from build123d import *

# Parameters (mm, degrees)
BOSS_EXTRUDE1_DEPTH = 3
SKETCH2_W           = 10
SKETCH2_H           = 3
SKETCH2_W_2         = 3
SKETCH2_H_2         = 12
CUT_EXTRUDE1_DEPTH  = 10
SKETCH5_R           = 1.7
SKETCH5_W           = 3
SKETCH5_H           = 5
CUT_EXTRUDE2_DEPTH  = 3
SKETCH6_R           = 2.5
SKETCH6_R_2         = 2.25
CUT_EXTRUDE3_DEPTH  = 10


with BuildPart() as part:
    # Sketch1 → Boss-Extrude1 (new body)
    with BuildSketch(Plane.XY.offset(152)):
        with BuildLine():
            Line((-82, 69.5), (82, 69.5))
            Line((82, 69.5), (82, 44))
            Line((82, 44), (88.6, 44))
            Line((88.6, 44), (88.6, 47))
            Line((88.6, 47), (93.6, 47))
            Line((93.6, 47), (93.6, 44))
            Line((93.6, 44), (98.6, 44))
            Line((98.6, 44), (98.6, 43.377104502))
            ThreePointArc((98.6, 43.377104502), (94.427800977, -13.668492876), (82, -69.5))
            Line((82, -69.5), (-82, -69.5))
            ThreePointArc((-82, -69.5), (-94.427800977, -13.668492876), (-98.6, 43.377104502))
            Line((-98.6, 43.377104502), (-98.6, 44))
            Line((-98.6, 44), (-93.6, 44))
            Line((-93.6, 44), (-93.6, 47))
            Line((-93.6, 47), (-88.6, 47))
            Line((-88.6, 47), (-88.6, 44))
            Line((-88.6, 44), (-82, 44))
            Line((-82, 44), (-82, 69.5))
        make_face()
    extrude(amount=BOSS_EXTRUDE1_DEPTH)

    # Sketch2 → Cut-Extrude1 (cut)
    with BuildSketch(Plane.XY.offset(155)):
        with Locations((0, 68)):
            Rectangle(SKETCH2_W, SKETCH2_H)
        with Locations((-22, 68)):
            Rectangle(SKETCH2_W, SKETCH2_H)
        with Locations((22, 68)):
            Rectangle(SKETCH2_W, SKETCH2_H)
        with Locations((-44, 68)):
            Rectangle(SKETCH2_W, SKETCH2_H)
        with Locations((44, 68)):
            Rectangle(SKETCH2_W, SKETCH2_H)
        with Locations((-66, 68)):
            Rectangle(SKETCH2_W, SKETCH2_H)
        with Locations((66, 68)):
            Rectangle(SKETCH2_W, SKETCH2_H)
        with Locations((-80.5, 53.5)):
            Rectangle(SKETCH2_W_2, SKETCH2_H_2)
        with Locations((80.5, 53.5)):
            Rectangle(SKETCH2_W_2, SKETCH2_H_2)
        with Locations((-80.5, 31.5)):
            Rectangle(SKETCH2_W_2, SKETCH2_H_2)
        with Locations((-80.5, 9.5)):
            Rectangle(SKETCH2_W_2, SKETCH2_H_2)
        with Locations((-80.5, -12.5)):
            Rectangle(SKETCH2_W_2, SKETCH2_H_2)
        with Locations((-80.5, -34.5)):
            Rectangle(SKETCH2_W_2, SKETCH2_H_2)
        with Locations((-80.5, -56.5)):
            Rectangle(SKETCH2_W_2, SKETCH2_H_2)
        with Locations((80.5, -56.5)):
            Rectangle(SKETCH2_W_2, SKETCH2_H_2)
        with Locations((80.5, -34.5)):
            Rectangle(SKETCH2_W_2, SKETCH2_H_2)
        with Locations((80.5, -12.5)):
            Rectangle(SKETCH2_W_2, SKETCH2_H_2)
        with Locations((80.5, 9.5)):
            Rectangle(SKETCH2_W_2, SKETCH2_H_2)
        with Locations((80.5, 31.5)):
            Rectangle(SKETCH2_W_2, SKETCH2_H_2)
    extrude(amount=-CUT_EXTRUDE1_DEPTH, mode=Mode.SUBTRACT)

    # Sketch5 → Cut-Extrude2 (cut)
    with BuildSketch(Plane.XY.offset(155)):
        with Locations((22.86677044, -57.9)):
            Circle(SKETCH5_R)
        with Locations((22.86677044, -34.5)):
            Circle(SKETCH5_R)
        Polygon((63.508529611, 46.5), (57.735026919, 56.5), (46.188021535, 56.5), (40.414518843, 46.5), (46.188021535, 36.5), (57.735026919, 36.5), align=None)
        Polygon((31.754264805, 41.5), (20.207259422, 41.5), (14.43375673, 31.5), (20.207259422, 21.5), (31.754264805, 21.5), (37.527767497, 31.5), align=None)
        Polygon((-20.207259422, 41.5), (-31.754264805, 41.5), (-37.527767497, 31.5), (-31.754264805, 21.5), (-20.207259422, 21.5), (-14.43375673, 31.5), align=None)
        Polygon((-20.207259422, 11.5), (-31.754264805, 11.5), (-37.527767497, 1.5), (-31.754264805, -8.5), (-20.207259422, -8.5), (-14.43375673, 1.5), align=None)
        Polygon((31.754264805, 11.5), (20.207259422, 11.5), (14.43375673, 1.5), (20.207259422, -8.5), (31.754264805, -8.5), (37.527767497, 1.5), align=None)
        Polygon((63.508529611, 16.5), (57.735026919, 26.5), (46.188021535, 26.5), (40.414518843, 16.5), (46.188021535, 6.5), (57.735026919, 6.5), align=None)
        Polygon((-20.207259422, -18.5), (-31.754264805, -18.5), (-37.527767497, -28.5), (-31.754264805, -38.5), (-20.207259422, -38.5), (-14.43375673, -28.5), align=None)
        Polygon((31.754264805, -18.5), (20.207259422, -18.5), (14.43375673, -28.5), (37.527767497, -28.5), align=None)
        Polygon((63.508529611, -13.5), (57.735026919, -3.5), (46.188021535, -3.5), (40.414518843, -13.5), (46.188021535, -23.5), (57.735026919, -23.5), align=None)
        Polygon((-20.207259422, -48.5), (-31.754264805, -48.5), (-37.527767497, -58.5), (-36.950417228, -59.5), (-15.011106999, -59.5), (-14.43375673, -58.5), align=None)
        Polygon((31.754264805, -48.5), (20.207259422, -48.5), (37.527767497, -58.5), align=None)
        Polygon((63.508529611, -43.5), (57.735026919, -33.5), (46.188021535, -33.5), (40.414518843, -43.5), (46.188021535, -53.5), (57.735026919, -53.5), align=None)
        Polygon((-40.412994616, 46.5), (-46.186497308, 56.5), (-57.733502692, 56.5), (-63.507005384, 46.5), (-57.733502692, 36.5), (-46.186497308, 36.5), align=None)
        Polygon((-40.412994616, 16.5), (-46.186497308, 26.5), (-57.733502692, 26.5), (-63.507005384, 16.5), (-57.733502692, 6.5), (-46.186497308, 6.5), align=None)
        Polygon((-40.412994616, -13.5), (-46.186497308, -3.5), (-57.733502692, -3.5), (-63.507005384, -13.5), (-57.733502692, -23.5), (-46.186497308, -23.5), align=None)
        Polygon((-40.412994616, -43.5), (-46.186497308, -33.5), (-57.733502692, -33.5), (-63.507005384, -43.5), (-57.733502692, -53.5), (-46.186497308, -53.5), align=None)
        with Locations((0, -62)):
            Rectangle(SKETCH5_W, SKETCH5_H)
    extrude(amount=-CUT_EXTRUDE2_DEPTH, mode=Mode.SUBTRACT)

    # Sketch6 → Cut-Extrude3 (cut)
    with BuildSketch(Plane.XY.offset(155)):
        with Locations((0, -52.5)):
            Circle(SKETCH6_R)
        with Locations((-7.25, -52.5)):
            Circle(SKETCH6_R_2)
        with Locations((7.25, -52.5)):
            Circle(SKETCH6_R_2)
    extrude(amount=-CUT_EXTRUDE3_DEPTH, mode=Mode.SUBTRACT)


solid = part.part
Geometry: final body of the model. Coordinates: model frame, mm. Give positions to 0.01 mm unless a question says otherwise; leave off trailing zeros. Write each loop counter-clockwise with the first axis right and the second up, starting at its lowest first coordinate (ties: lowest second). Pieces come first, ordered by that corner, then holes. Notation, with made-up numbers: (-38.75, 17) - (8.25, 17) arc R28 cw to (8.25, 42) - close; hole circle Ø4 at (-14, 56.25). An arc over 180 degrees is marked (long way). Return JSON: item names as keys, results as strings. Group by question number.
1) First-contact query: P1, Ø0.9, axis at y = 8.5, z = 154, coming from the -X side; P2, Ø10, axis at x = -23.5, y = -20.5, coming from the +Z side; P3, Ø1.5, axis at y = -34.5, z = 154, coming from the -X side; P4, Ø0.9, axis at y = 67.5, z = 153.5, coming from the -X side. Flat tips, straight axial feed; report the tip coordinate or a pass-through.
2) Section B-B on z = 153.65. State how many separate pieces and enclosed holes the cut face has, plus the area to 3 significant figures.
3) Line query: line 1 (Y direction, x = 0, z = 153.95); line 2 (Y direction, x = -58.5, z = 154.6); line 3 (X direction, y = 4.5, z = 153.4). Output: solid intervals per line, ascending.
4) Mould query, pull axis X, two halves, no side actions, for faces 1 (the flat face through (1, 1, 152)), 2 (the cylindrical face through (6.96, -50.27, 153.52)). Classes: released by +X, released by -X, zero draft, split by the parting line, or undercut.
5) Section A-A on x = 7.25. Return the cut outline in (y, z).
Filled in:
{
 "1": {"P1": "stops at x = -97.09", "P2": "stops at z = 155", "P3": "stops at x = -90.94", "P4": "stops at x = -82"},
 "2": {"separate pieces": "1", "enclosed holes": "32", "area": "19,700 mm^2"},
 "3": {"line 1": "y = -69.5 to -64.5, -59.5 to -55, -50 to 66.5", "line 2": "y = -69.5 to -52.17, -34.83 to -22.17, -4.83 to 7.83, 25.17 to 37.83, 55.17 to 69.5", "line 3": "x = -96.67 to -82, -79 to -35.8, -16.17 to 16.17, 35.8 to 79, 82 to 96.67"},
 "4": {"face 1": "zero draft", "face 2": "undercut"},
 "5": {"outline": "(-69.5, 152) - (-54.75, 152) - (-54.75, 155) - (-69.5, 155) - close; (-50.25, 152) - (69.5, 152) - (69.5, 155) - (-50.25, 155) - close"}
}
